For this review, take the finished solid that the model builds, in its own axes (mm). Face numbers are marked on the shaded views. A direction names the side the tool comes from. Coordinates: 2 decimals unless noted, no trailing zeros. Order: outer loops, then holes, each group sorted by start corner. A loop starts at its lowest first (then second) coordinate and runs counter-clockwise, first axis right, second up. Notation, with made-up numbers: (46.5, -17) - (58.5, -17) arc R17 cw to (58.5, -13) - close; hole circle Ø11 at (27, 18). An arc over 180 degrees is marked (long way). One line per item, written item: value. Start each with the question number.
(1) Consider section A-A on z = 9. Write out the cut boundary in (x, y), then the cut area to 3 significant figures.
(2) Consider section B-B on y = 19. Write out the cut boundary in (x, z).
(3) For the marked faces 4 and 5, list the 3-axis set-ups (+Z, -Z, +X, -X, +Y, -Y) from which the entire face can be reached by the end or side of a thin tool; tool diameter is ignored.
(4) Mouldability with a two-part tool opening along Y and no side actions: class the marked faces 1, 2 and 3 as released by +Y, released by -Y, zero draft, split by the parting line, or undercut.
(5) To check wall thickness, follow line 1 along Y through (x, z) = (6, 23); line 2 along X through (y, z) = (-17, 24); line 3 along Z through (x, y) = (35, -2). State the ranges of each line that lie inside material, in increasing order.
(6) Consider section C-C on x = -8. Write out the cut boundary in (y, z).
(7) Clearance check with a flat-ended pin moving along its axis: pin 1 (1.5 mm diameter, centred on x = 7.5, y = -17, fed in from -Z). State where the tip first meets the part, or that it passes through.
```python
from build123d import *

# Parameters (mm, degrees)
BOSS_EXTRUDE1_DEPTH = 46
BOSS_EXTRUDE2_DEPTH = 1.5
CHAMFER1_SIZE       = 1.5


with BuildPart() as part:
    # Sketch1 → Boss-Extrude1 (new body)
    with BuildSketch(Plane.XY):
        with BuildLine():
            Line((-30.297360891, 123.437225034), (-45.325625095, 81.692046689))
            ThreePointArc((-45.325625095, 81.692046689), (-45.904954257, 79.506966326), (-46.1, 77.254821654))
            Line((-46.1, 77.254821654), (-46.1, -60.733642247))
            ThreePointArc((-46.1, -60.733642247), (-42.263098834, -69.99674108), (-33, -73.833642247))
            Line((-33, -73.833642247), (33, -73.833642247))
            ThreePointArc((33, -73.833642247), (42.263098834, -69.99674108), (46.1, -60.733642247))
            Line((46.1, -60.733642247), (46.1, 77.254821654))
            ThreePointArc((46.1, 77.254821654), (45.904954257, 79.506966326), (45.325625095, 81.692046689))
            Line((45.325625095, 81.692046689), (30.297360891, 123.437225034))
            ThreePointArc((30.297360891, 123.437225034), (25.504409692, 129.717687436), (17.971735796, 132.1))
            Line((17.971735796, 132.1), (-17.971735796, 132.1))
            ThreePointArc((-17.971735796, 132.1), (-25.504409692, 129.717687436), (-30.297360891, 123.437225034))
        make_face()
        with BuildLine():
            Line((-27.474698655, 122.42106663), (-42.50296286, 80.675888284))
            ThreePointArc((-42.50296286, 80.675888284), (-42.949621221, 78.991208005), (-43.1, 77.254821654))
            Line((-43.1, 77.254821654), (-43.1, -60.733642247))
            ThreePointArc((-43.1, -60.733642247), (-40.14177849, -67.875420737), (-33, -70.833642247))
            Line((-33, -70.833642247), (33, -70.833642247))
            ThreePointArc((33, -70.833642247), (40.14177849, -67.875420737), (43.1, -60.733642247))
            Line((43.1, -60.733642247), (43.1, 77.254821654))
            ThreePointArc((43.1, 77.254821654), (42.949621221, 78.991208005), (42.50296286, 80.675888284))
            Line((42.50296286, 80.675888284), (27.474698655, 122.42106663))
            ThreePointArc((27.474698655, 122.42106663), (23.779369868, 127.263255199), (17.971735796, 129.1))
            Line((17.971735796, 129.1), (-17.971735796, 129.1))
            ThreePointArc((-17.971735796, 129.1), (-23.779369868, 127.263255199), (-27.474698655, 122.42106663))
        make_face(mode=Mode.SUBTRACT)
    extrude(amount=BOSS_EXTRUDE1_DEPTH)

    # Sketch2 → Boss-Extrude2 (add)
    with BuildSketch(Plane.XY.offset(46)):
        with BuildLine():
            Line((17.971735796, 132.1), (-17.971735796, 132.1))
            ThreePointArc((-17.971735796, 132.1), (-25.504409692, 129.717687436), (-30.297360891, 123.437225034))
            Line((-30.297360891, 123.437225034), (-45.325625095, 81.692046689))
            ThreePointArc((-45.325625095, 81.692046689), (-45.904954257, 79.506966326), (-46.1, 77.254821654))
            Line((-46.1, 77.254821654), (-46.1, -60.733642247))
            ThreePointArc((-46.1, -60.733642247), (-42.263098834, -69.99674108), (-33, -73.833642247))
            Line((-33, -73.833642247), (33, -73.833642247))
            ThreePointArc((33, -73.833642247), (42.263098834, -69.99674108), (46.1, -60.733642247))
            Line((46.1, -60.733642247), (46.1, 77.254821654))
            ThreePointArc((46.1, 77.254821654), (45.904954257, 79.506966326), (45.325625095, 81.692046689))
            Line((45.325625095, 81.692046689), (30.297360891, 123.437225034))
            ThreePointArc((30.297360891, 123.437225034), (25.504409692, 129.717687436), (17.971735796, 132.1))
        make_face()
    extrude(amount=BOSS_EXTRUDE2_DEPTH)

    # Chamfer1
    chamfer1_edges = [part.edges().sort_by_distance(p)[0] for p in [
        (-23.779369868, 127.263255199, 0),
        (-34.988830758, 101.548477457, 0),
        (-42.949621221, 78.991208005, 0),
        (-43.1, 8.260589704, 0),
        (-40.14177849, -67.875420737, 0),
        (0, -70.833642247, 0),
        (40.14177849, -67.875420737, 0),
        (43.1, 8.260589704, 0),
        (42.949621221, 78.991208005, 0),
        (34.988830758, 101.548477457, 0),
        (23.779369868, 127.263255199, 0),
        (0, 129.1, 0),
        (25.504409692, 129.717687436, 47.5),
        (0, 132.1, 47.5),
        (-25.504409692, 129.717687436, 47.5),
        (-37.811492993, 102.564635861, 47.5),
        (-45.904954257, 79.506966326, 47.5),
        (-46.1, 8.260589704, 47.5),
        (-42.263098834, -69.99674108, 47.5),
        (0, -73.833642247, 47.5),
        (42.263098834, -69.99674108, 47.5),
        (46.1, 8.260589704, 47.5),
        (45.904954257, 79.506966326, 47.5),
        (37.811492993, 102.564635861, 47.5),
    ]]
    chamfer(chamfer1_edges, length=CHAMFER1_SIZE)


solid = part.part
```
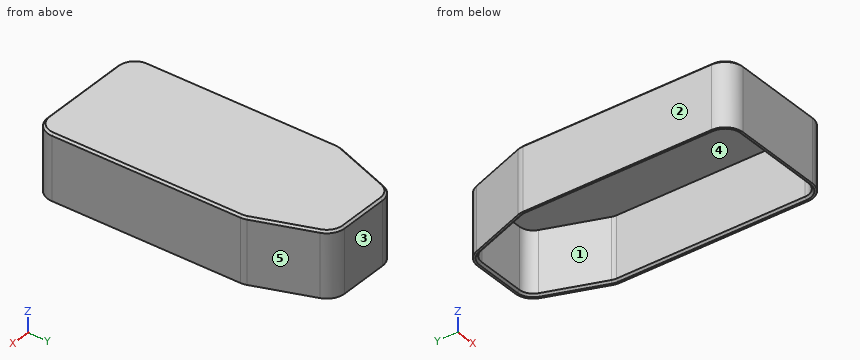
Geometry check:
1. outline: (-46.1, -60.73) arc R13.1 ccw to (-33, -73.83) - (33, -73.83) arc R13.1 ccw to (46.1, -60.73) - (46.1, 77.25) arc R13.1 ccw to (45.33, 81.69) - (30.3, 123.44) arc R13.1 ccw to (17.97, 132.1) - (-17.97, 132.1) arc R13.1 ccw to (-30.3, 123.44) - (-45.33, 81.69) arc R13.1 ccw to (-46.1, 77.25) - close; hole (-43.1, -60.73) arc R10.1 ccw to (-33, -70.83) - (33, -70.83) arc R10.1 ccw to (43.1, -60.73) - (43.1, 77.25) arc R10.1 ccw to (42.5, 80.68) - (27.47, 122.42) arc R10.1 ccw to (17.97, 129.1) - (-17.97, 129.1) arc R10.1 ccw to (-27.47, 122.42) - (-42.5, 80.68) arc R10.1 ccw to (-43.1, 77.25) - close
1. area: 1,620 mm^2
2. outline: (-46.1, 0) - (-44.6, 0) - (-43.1, 1.5) - (-43.1, 46) - (43.1, 46) - (43.1, 1.5) - (44.6, 0) - (46.1, 0) - (46.1, 46) - (44.6, 47.5) - (-44.6, 47.5) - (-46.1, 46) - close
3. face 4: -Z
3. face 5: +Z, -Z, +X, +Y
4. face 1: undercut
4. face 2: zero draft
4. face 3: released by +Y
5. line 1: y = -73.83 to -70.83, 129.1 to 132.1
5. line 2: x = -46.1 to -43.1, 43.1 to 46.1
5. line 3: z = 46 to 47.5
6. outline: (-73.83, 0) - (-72.33, 0) - (-70.83, 1.5) - (-70.83, 46) - (129.1, 46) - (129.1, 1.5) - (130.6, 0) - (132.1, 0) - (132.1, 46) - (130.6, 47.5) - (-72.33, 47.5) - (-73.83, 46) - close
7. pin 1: stops at z = 46
